Solid Edge part; units mm, degrees
sketch "Sketch1" plane through (0, 0, 0) normal (0, 0, 1) x (1, 0, 0)
  line L0 (-25.4, 19.05) -> (25.4, 19.05)
  line L1 (25.4, 19.05) -> (25.4, 12.7)
  line L2 (25.4, 12.7) -> (9.525, 12.7)
  line L3 (9.525, 12.7) -> (9.525, -12.7)
  line L4 (9.525, -12.7) -> (-9.525, -12.7)
  line L5 (-9.525, -12.7) -> (-9.525, 12.7)
  line L6 (-9.525, 12.7) -> (-25.4, 12.7)
  line L7 (-25.4, 12.7) -> (-25.4, 19.05)
  dimension "D1" = 25.4
  dimension "D2" = 9.525
  dimension "D3" = 25.4
  dimension "D4" = 25.4
  dimension "D5" = 9.525
  dimension "D6" = 9.525
  dimension "D7" = 25.4
  dimension "D8" = 9.525
extrude "Protrusion1" add sketch "Sketch1" along normal blind 12.7
fillet "Round_1" radius 3.175 6 edges at (9.525, 12.7, 6.35) (9.525, -12.7, 6.35) (-9.525, -12.7, 6.35) (25.4, 12.7, 6.35) (-9.525, 12.7, 6.35) (-25.4, 12.7, 6.35)
sketch "Sketch2" plane through (0, 3.175, 12.7) normal (0, 0, 1) x (0, 1, 0)
  circle A0 centre (-3.175, 0) radius 6.35
extrude "PivotHole" cut sketch "Sketch2" against normal blind 10.16
sketch "Sketch3" plane through (-17.4625, 12.7, 6.35) normal (0, -1, 0) x (1, 0, 0)
  circle A0 centre (-0.3175, 0) radius 3.175
  dimension "D1" = 0.3175
extrude "v_1" cut sketch "Sketch3" against normal blind 25.4
mirror "Mirror1" about plane through (0, 0, 0) normal (1, 0, 0) of "v_1"
properties material "Aluminum, 6061-T6"
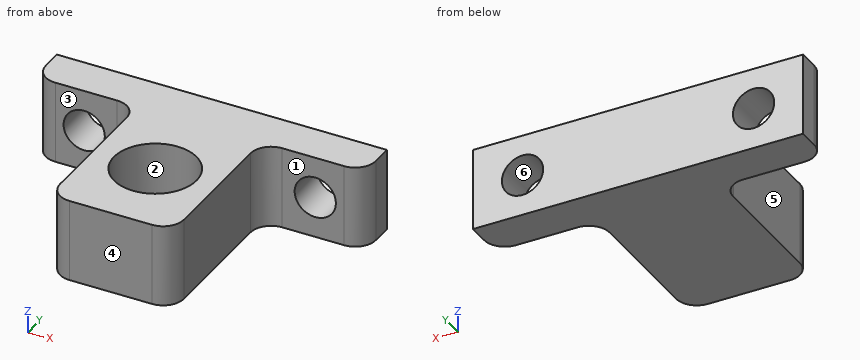
The model under review builds one solid part; all positions refer to its coordinate system, in mm. Face numbers are marked on the shaded views. A direction names the side the tool comes from. Coordinates: 2 decimals unless noted, no trailing zeros. Write each loop counter-clockwise with the first axis right and the second up, starting at its lowest first coordinate (ties: lowest second). Pieces come first, ordered by that corner, then holes. Notation, with made-up numbers: (-27.75, 69.25) - (26.25, 69.25) arc R15 ccw to (26.25, 84.25) - close; hole circle Ø4 at (49.25, 44). An arc over 180 degrees is marked (long way). Write item = value, one per line.
(1) Consider section B-B, the plane x = -17.78. Give the boundary of the cut face in (y, z) (3 decimals), then the cut area to 3 significant figures.
Result sheet:
outline = (12.7, 0) - (19.05, 0) - (19.05, 3.175) - (12.7, 3.175) - close; (12.7, 9.525) - (19.05, 9.525) - (19.05, 12.7) - (12.7, 12.7) - close
area = 40.3 mm^2
(2) Consider section A-A, the plane z = 6.35. Give the boundary of the cut face in (x, y) (3 decimals).
Result sheet:
outline = (-25.4, 15.875) arc R3.175 ccw to (-22.225, 12.7) - (-20.955, 12.7) - (-20.955, 19.05) - (-25.4, 19.05) - close; (-14.605, 12.7) - (-12.7, 12.7) arc R3.175 cw to (-9.525, 9.525) - (-9.525, -9.525) arc R3.175 ccw to (-6.35, -12.7) - (6.35, -12.7) arc R3.175 ccw to (9.525, -9.525) - (9.525, 9.525) arc R3.175 cw to (12.7, 12.7) - (14.605, 12.7) - (14.605, 19.05) - (-14.605, 19.05) - close; (20.955, 12.7) - (22.225, 12.7) arc R3.175 ccw to (25.4, 15.875) - (25.4, 19.05) - (20.955, 19.05) - close; hole circle Ø12.7 at (0, 0)
(3) For P1, Ø3, axis at x = 16.5, z = 3.5, coming from the -Y side; P2, Ø2, axis at y = 2, z = 10, coming from the +X side (3 decimals); P3, Ø16.5, axis at x = 0, y = 0, coming from the +Z side; P4, Ø4, axis at y = 7.5, z = 7.5, coming from the -X side (3 decimals), all flat-tipped, find the tip position at first contact; note any pin that passes through.
Result sheet:
P1 = 12.7
P2 = 9.525
P3 = 12.7
P4 = -9.525
(4) Consider section C-C, the plane y = 16.5. Give the boundary of the cut face in (x, z) (3 decimals), then the cut area to 3 significant figures.
Result sheet:
outline = (-25.4, 0) - (25.4, 0) - (25.4, 12.7) - (-25.4, 12.7) - close; hole circle Ø6.35 at (-17.78, 6.35); hole circle Ø6.35 at (17.78, 6.35)
area = 582 mm^2
(5) For line 1 (X direction, y = 0, z = 5.5) (3 decimals); line 2 (Z direction, x = -17.78, y = 17.75) (3 decimals); line 3 (X direction, y = -6.5, z = 11) (3 decimals), list the stretches that pass through material, from the lowest coordinate up. Write a range as [from, to].
Result sheet:
line_1 = [-9.525, -6.35], [6.35, 9.525]
line_2 = [0, 3.175], [9.525, 12.7]
line_3 = [-9.525, 9.525]
(6) Machinability: for the marked faces 1, 2 and 3, which of the approach directions +Z, -Z, +X, -X, +Y, -Y give a long, thin tool a straight path to every point of the face, cutting with its end or side? Answer none if there is none.
Result sheet:
face_1 = +Z, -Z, +X, -Y
face_2 = +Z
face_3 = +Z, -Z, -X, -Y
(7) Mouldability with a two-part tool opening along X and no side actions: class the marked faces 4, 5 and 6 as pulls with the +X half, pulls with the -X half, needs draft (parallel to the pull), parting line crosses it, or undercut.
Result sheet:
face_4 = needs draft
face_5 = pulls with the -X half
face_6 = undercut
(8) Consider section D-D, the plane x = 0. Give the boundary of the cut face in (y, z).
Result sheet:
outline = (-12.7, 0) - (19.05, 0) - (19.05, 12.7) - (6.35, 12.7) - (6.35, 2.54) - (-6.35, 2.54) - (-6.35, 12.7) - (-12.7, 12.7) - close
